```python
from build123d import *

# Parameters (mm, degrees)
F0_R     = 3
F0_R_2   = 2.5
F1_DEPTH = 490
F2_R     = 2
F3_R     = 7


# Not quite as in the source:
# - a feature names something its author has since deleted; it is built from what else it names


with BuildPart() as f1:
    # F0 (on Top) → F1 (new body)
    with BuildSketch(Plane.XY):
        with BuildLine():
            Line((18.15, -30), (30, -30))
            Line((30, -30), (30, -18.15))
            Line((30, -18.15), (27.5, -18.15))
            Line((27.5, -18.15), (27.5, -20.15))
            Line((27.5, -20.15), (21.5477069044, -20.15))
            ThreePointArc((21.5477069044, -20.15), (19.5, -15), (21.5477069044, -9.85))
            Line((21.5477069044, -9.85), (27.5, -9.85))
            Line((27.5, -9.85), (27.5, -11.85))
            Line((27.5, -11.85), (30, -11.85))
            Line((30, -11.85), (30, 11.85))
            Line((30, 11.85), (27.5, 11.85))
            Line((27.5, 11.85), (27.5, 9.85))
            Line((27.5, 9.85), (21.5477069044, 9.85))
            ThreePointArc((21.5477069044, 9.85), (19.5, 15), (21.5477069044, 20.15))
            Line((21.5477069044, 20.15), (27.5, 20.15))
            Line((27.5, 20.15), (27.5, 18.15))
            Line((27.5, 18.15), (30, 18.15))
            Line((30, 18.15), (30, 30))
            Line((30, 30), (18.15, 30))
            Line((18.15, 30), (18.15, 27.5))
            Line((18.15, 27.5), (20.15, 27.5))
            Line((20.15, 27.5), (20.15, 21.5477069044))
            ThreePointArc((20.15, 21.5477069044), (15, 19.5), (9.85, 21.5477069044))
            Line((9.85, 21.5477069044), (9.85, 27.5))
            Line((9.85, 27.5), (11.85, 27.5))
            Line((11.85, 27.5), (11.85, 30))
            Line((11.85, 30), (-11.85, 30))
            Line((-11.85, 30), (-11.85, 27.5))
            Line((-11.85, 27.5), (-9.85, 27.5))
            Line((-9.85, 27.5), (-9.85, 21.5477069044))
            ThreePointArc((-9.85, 21.5477069044), (-15, 19.5), (-20.15, 21.5477069044))
            Line((-20.15, 21.5477069044), (-20.15, 27.5))
            Line((-20.15, 27.5), (-18.15, 27.5))
            Line((-18.15, 27.5), (-18.15, 30))
            Line((-18.15, 30), (-30, 30))
            Line((-30, 30), (-30, 18.15))
            Line((-30, 18.15), (-27.5, 18.15))
            Line((-27.5, 18.15), (-27.5, 20.15))
            Line((-27.5, 20.15), (-21.5477069044, 20.15))
            ThreePointArc((-21.5477069044, 20.15), (-19.5, 15), (-21.5477069044, 9.85))
            Line((-21.5477069044, 9.85), (-27.5, 9.85))
            Line((-27.5, 9.85), (-27.5, 11.85))
            Line((-27.5, 11.85), (-30, 11.85))
            Line((-30, 11.85), (-30, -11.85))
            Line((-30, -11.85), (-27.5, -11.85))
            Line((-27.5, -11.85), (-27.5, -9.85))
            Line((-27.5, -9.85), (-21.5477069044, -9.85))
            ThreePointArc((-21.5477069044, -9.85), (-19.5, -15), (-21.5477069044, -20.15))
            Line((-21.5477069044, -20.15), (-27.5, -20.15))
            Line((-27.5, -20.15), (-27.5, -18.15))
            Line((-27.5, -18.15), (-30, -18.15))
            Line((-30, -18.15), (-30, -30))
            Line((-30, -30), (-18.15, -30))
            Line((-18.15, -30), (-18.15, -27.5))
            Line((-18.15, -27.5), (-20.15, -27.5))
            Line((-20.15, -27.5), (-20.15, -21.5477069044))
            ThreePointArc((-20.15, -21.5477069044), (-15, -19.5), (-9.85, -21.5477069044))
            Line((-9.85, -21.5477069044), (-9.85, -27.5))
            Line((-9.85, -27.5), (-11.85, -27.5))
            Line((-11.85, -27.5), (-11.85, -30))
            Line((-11.85, -30), (11.85, -30))
            Line((11.85, -30), (11.85, -27.5))
            Line((11.85, -27.5), (9.85, -27.5))
            Line((9.85, -27.5), (9.85, -21.5477069044))
            ThreePointArc((9.85, -21.5477069044), (15, -19.5), (20.15, -21.5477069044))
            Line((20.15, -21.5477069044), (20.15, -27.5))
            Line((20.15, -27.5), (18.15, -27.5))
            Line((18.15, -27.5), (18.15, -30))
        make_face()
        with Locations((-25, -25)):
            Circle(F0_R, mode=Mode.SUBTRACT)
        with Locations((-15, -15)):
            Circle(F0_R_2, mode=Mode.SUBTRACT)
        with Locations((25, -25)):
            Circle(F0_R, mode=Mode.SUBTRACT)
        with Locations((15, -15)):
            Circle(F0_R_2, mode=Mode.SUBTRACT)
        with Locations((-25, 25)):
            Circle(F0_R, mode=Mode.SUBTRACT)
        with Locations((-15, 15)):
            Circle(F0_R_2, mode=Mode.SUBTRACT)
        Polygon((-7, 22), (-7, 27.5), (0, 27.5), (7, 27.5), (7, 22), (10, 16), (10, 10), (16, 10), (22, 7), (27.5, 7), (27.5, 0), (27.5, -7), (22, -7), (16, -10), (10, -10), (10, -16), (7, -22), (7, -27.5), (0, -27.5), (-7, -27.5), (-7, -22), (-10, -16), (-10, -10), (-16, -10), (-22, -7), (-27.5, -7), (-27.5, 0), (-27.5, 7), (-22, 7), (-16, 10), (-10, 10), (-10, 16), align=None, mode=Mode.SUBTRACT)
        with Locations((15, 15)):
            Circle(F0_R_2, mode=Mode.SUBTRACT)
        with Locations((25, 25)):
            Circle(F0_R, mode=Mode.SUBTRACT)
    extrude(amount=F1_DEPTH)

    # F2
    f2_edges = [f1.edges().sort_by_distance(p)[0] for p in [
        (-7, 27.5, 245),
        (7, 27.5, 245),
    ]]
    fillet(f2_edges, radius=F2_R)

    # F3
    f3_edges = [f1.edges().sort_by_distance(p)[0] for p in [
        (-10, 16, 245),
        (10, 16, 245),
    ]]
    fillet(f3_edges, radius=F3_R)


solid = f1.part
```
Input: part model. Units: mm. Frame: model coordinates. A direction names the side the tool comes from. Give positions to 0.01 mm unless a question says otherwise; leave off trailing zeros. Loops run counter-clockwise (first coordinate to the right, second up) from the corner with the lowest first, then second, coordinate; pieces in that order, holes last.
1) Reachability of faces 1 (the flat face through (30, -24, 242)), 2 (the cylindrical face through (-14.9, 19.5, 241.6)) from +Z, -Z, +X, -X, +Y, -Y: full face, straight path, thin tool, end or side. Return the list, or none.
A:
face 1: +Z, -Z, +X, +Y, -Y
face 2: +Z, -Z
2) Mould query, pull axis X, two halves, no side actions, for faces 3 (the cylindrical face through (-19.5, 15.1, 241.6)), 4 (the flat face through (30, 24, 242)), 5 (the flat face through (11, -11, 490)). Classes: released by +X, released by -X, zero draft, split by the parting line, or undercut.
A:
face 3: undercut
face 4: released by +X
face 5: zero draft
3) Section query B-B on z = 117. Count the separate pieces of the cut face and the enclosed holes in it, and give its area (3 significant figures).
A:
separate pieces: 1
enclosed holes: 9
area: 1,080 mm2
4) Section query A-A on y = 1.5. Return the cut outline in (x, z).
A:
outline: (-30, 0) - (-27.5, 0) - (-27.5, 490) - (-30, 490) - close; (27.5, 0) - (30, 0) - (30, 490) - (27.5, 490) - close
5) Line query: L1, parallel to Y at x = -15, z = 244; L2, parallel to X at y = 23.5, z = 183; L3, parallel to X at y = -6, z = 460. Output: solid intervals per line, ascending.
A:
L1: y = -19.5 to -17.5, -12.5 to -10, 10 to 12.5, 17.5 to 19.5
L2: x = -30 to -27.6, -22.4 to -20.15, -9.85 to -7, 7 to 9.85, 20.15 to 22.4, 27.6 to 30
L3: x = -30 to -27.5, 27.5 to 30
